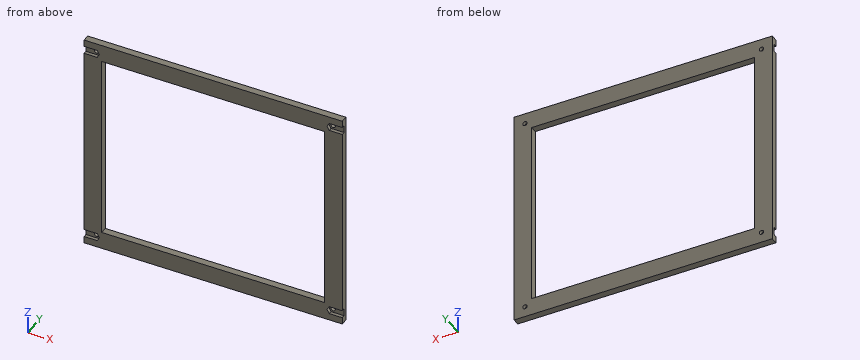
from build123d import *

# Parameters (mm, degrees)
SKETCH2_W           = 165
SKETCH2_H           = 140
BOSS_EXTRUDE1_DEPTH = 5
SKETCH2_3_R         = 1.6
SKETCH2_3_W         = 3
SKETCH2_3_H         = 5.7
BOSS_EXTRUDE2_DEPTH = 2.5


with BuildPart() as part:
    # Sketch2 → Boss-Extrude1 (new body)
    with BuildSketch(Plane(origin=(0, 0, 0), x_dir=(1, 0, 0), z_dir=(0, 1, 0))):
        Polygon((-95.5, -77.85), (-95.5, -83), (95.5, -83), (95.5, -77.85), (85.854551733, -77.85), (84.209103466, -75), (85.854551733, -72.15), (95.5, -72.15), (95.5, 72.15), (85.854551733, 72.15), (84.209103466, 75), (85.854551733, 77.85), (95.5, 77.85), (95.5, 83), (-95.5, 83), (-95.5, 77.85), (-85.854551733, 77.85), (-84.209103466, 75), (-85.854551733, 72.15), (-95.5, 72.15), (-95.5, -72.15), (-85.854551733, -72.15), (-84.209103466, -75), (-85.854551733, -77.85), align=None)
        Rectangle(SKETCH2_W, SKETCH2_H, mode=Mode.SUBTRACT)
    extrude(amount=-BOSS_EXTRUDE1_DEPTH)

    # Sketch2_3 → Boss-Extrude2 (add)
    with BuildSketch(Plane(origin=(0, 0, 0), x_dir=(1, 0, 0), z_dir=(0, 1, 0))):
        Polygon((-85.854551733, 77.85), (-89.145448267, 77.85), (-90.790896534, 75), (-89.145448267, 72.15), (-85.854551733, 72.15), (-84.209103466, 75), align=None)
        with Locations((-87.5, 75)):
            Circle(SKETCH2_3_R, mode=Mode.SUBTRACT)
        Polygon((-90.790896534, -75), (-89.145448267, -72.15), (-85.854551733, -72.15), (-84.209103466, -75), (-85.854551733, -77.85), (-89.145448267, -77.85), align=None)
        with Locations((-87.5, -75)):
            Circle(SKETCH2_3_R, mode=Mode.SUBTRACT)
        Polygon((85.854551733, -77.85), (89.145448267, -77.85), (90.790896534, -75), (89.145448267, -72.15), (85.854551733, -72.15), (84.209103466, -75), align=None)
        with Locations((87.5, -75)):
            Circle(SKETCH2_3_R, mode=Mode.SUBTRACT)
        Polygon((90.790896534, 75), (89.145448267, 72.15), (85.854551733, 72.15), (84.209103466, 75), (85.854551733, 77.85), (89.145448267, 77.85), align=None)
        with Locations((87.5, 75)):
            Circle(SKETCH2_3_R, mode=Mode.SUBTRACT)
        Polygon((89.145448267, 72.15), (92.5, 72.15), (92.5, 77.85), (89.145448267, 77.85), (90.790896534, 75), align=None)
        Polygon((89.145448267, -77.85), (92.5, -77.85), (92.5, -72.15), (89.145448267, -72.15), (90.790896534, -75), align=None)
        Polygon((-92.5, -72.15), (-92.5, -77.85), (-89.145448267, -77.85), (-90.790896534, -75), (-89.145448267, -72.15), align=None)
        Polygon((-92.5, 77.85), (-92.5, 72.15), (-89.145448267, 72.15), (-90.790896534, 75), (-89.145448267, 77.85), align=None)
        with Locations((-94, 75)):
            Rectangle(SKETCH2_3_W, SKETCH2_3_H)
        with Locations((-94, -75)):
            Rectangle(SKETCH2_3_W, SKETCH2_3_H)
        with Locations((94, -75)):
            Rectangle(SKETCH2_3_W, SKETCH2_3_H)
        with Locations((94, 75)):
            Rectangle(SKETCH2_3_W, SKETCH2_3_H)
    extrude(amount=-BOSS_EXTRUDE2_DEPTH)


solid = part.part
Design review of the part built by this model. Coordinates are the model's own, in mm. Give positions to 0.01 mm unless a question says otherwise; leave off trailing zeros. Order: outer loops, then holes, each group sorted by start corner. A loop starts at its lowest first (then second) coordinate and runs counter-clockwise, first axis right, second up.
1. Add section B-B, the plane x = 68.5. State the section outline as (y, z) points, then the cut area to 3 significant figures.
Solution:
outline: (-5, -83) - (0, -83) - (0, -70) - (-5, -70) - close; (-5, 70) - (0, 70) - (0, 83) - (-5, 83) - close
area: 130 mm2
2. To check wall thickness, follow L1, parallel to Z at x = -87.5, y = -0.7; L2, parallel to X at y = -1.5, z = 75; L3, parallel to Z at x = -56, y = -2.15. State the ranges of each line that lie inside material, in increasing order.
Solution:
L1: z = -83 to -76.6, -73.4 to 73.4, 76.6 to 83
L2: x = -95.5 to -89.1, -85.9 to 85.9, 89.1 to 95.5
L3: z = -83 to -70, 70 to 83
3. Add section A-A, the plane y = -3.75. State the section outline as (x, z) points.
Solution:
outline: (-95.5, -83) - (95.5, -83) - (95.5, -77.85) - (85.85, -77.85) - (84.21, -75) - (85.85, -72.15) - (95.5, -72.15) - (95.5, 72.15) - (85.85, 72.15) - (84.21, 75) - (85.85, 77.85) - (95.5, 77.85) - (95.5, 83) - (-95.5, 83) - (-95.5, 77.85) - (-85.85, 77.85) - (-84.21, 75) - (-85.85, 72.15) - (-95.5, 72.15) - (-95.5, -72.15) - (-85.85, -72.15) - (-84.21, -75) - (-85.85, -77.85) - (-95.5, -77.85) - close; hole (-82.5, -70) - (82.5, -70) - (82.5, 70) - (-82.5, 70) - close
4. For pin 1 Ø3.5 at (x, z) = (-87.5, 75) entering from -Y, flat-tipped, find the tip position at first contact; note if it passes through.
Solution:
pin 1: stops at y = -2.5
5. Add section C-C, the plane z = 33.5. State the section outline as (x, y) points, then the cut area to 3 significant figures.
Solution:
outline: (-95.5, -5) - (-82.5, -5) - (-82.5, 0) - (-95.5, 0) - close; (82.5, -5) - (95.5, -5) - (95.5, 0) - (82.5, 0) - close
area: 130 mm2
